Input: part model. Units: mm. Frame: model coordinates. Give positions to 0.01 mm unless a question says otherwise; leave off trailing zeros. Order: outer loops, then holes, each group sorted by start corner. A loop starts at its lowest first (then second) coordinate and runs counter-clockwise, first axis right, second up. Notation, with made-up numbers: (14.25, -11.5) -> (52.25, -11.5) arc R24 cw to (52.25, 17.5) -> close; hole circle Ø1 at (62, 41.25). An arc over 180 degrees is marked (long way). Use a Markdown table: item, result. Add a question column.
from build123d import *

# Parameters (mm, degrees)
F0_R     = 7.1501
F0_R_2   = 6.227401
F1_DEPTH = 4.7498


with BuildPart() as f1:
    # F0 (on Front) → F1 (new body)
    with BuildSketch(Plane.XZ):
        with BuildLine():
            Line((-139.7, -25.4), (139.7, -25.4))
            ThreePointArc((139.7, -25.4), (162.15064, -16.10064), (171.45, 6.35))
            Line((171.45, 6.35), (171.45, 19.05))
            ThreePointArc((171.45, 19.05), (169.590128, 23.540128), (165.1, 25.4))
            Line((165.1, 25.4), (-165.1, 25.4))
            ThreePointArc((-165.1, 25.4), (-169.590128, 23.540128), (-171.45, 19.05))
            Line((-171.45, 19.05), (-171.45, 6.35))
            ThreePointArc((-171.45, 6.35), (-162.15064, -16.10064), (-139.7, -25.4))
        make_face()
        with Locations((-101.6, -12.7)):
            Circle(F0_R, mode=Mode.SUBTRACT)
        with Locations((101.6, -12.7)):
            Circle(F0_R, mode=Mode.SUBTRACT)
        with Locations((-152.4, 7.62)):
            Circle(F0_R_2, mode=Mode.SUBTRACT)
        with Locations((152.4, 7.62)):
            Circle(F0_R_2, mode=Mode.SUBTRACT)
    extrude(amount=F1_DEPTH)


solid = f1.part
Q1. Ray query, line 1 (X direction, y = -0.4, z = 3); line 2 (X direction, y = -2.2, z = -13.5); line 3 (Z direction, x = -101.6, y = -2.8). Return the intervals inside material, ascending.
Q2. Section query A-A (y = -3.2). Return loops of the section in (x, z), plus the area to 3 significant figures.
Q3. Section query D-D (x = 152.4). Return loops of the section in (y, z).
Q4. Section query B-B (x = 101.6). Return loops of the section in (y, z), plus the area to 3 significant figures.
Q5. Draft query along X for faces 1 (the cylindrical face through (-169.54, -2.34, 23.59)), 2 (the flat face through (-2, -4.75, 0)), 3 (the cylindrical face through (-94.78, -2.34, -10.55)). Return one class per face: +X half, -X half, draft (parallel to the pull), parting line (faces both ways), or undercut.
Q6. Section query C-C (z = -9). Return loops of the section in (x, y), plus the area to 3 significant figures.
Q7. First-contact query: pin 1 (2 mm diameter, centred on y = -2, z = -14.5, fed in from -X). Flat tip, straight axial feed; report the tip coordinate or a pass-through.
Solution:
| question | item | result |
|---|---|---|
| 1 | line 1 | x = -171.27 to -156.58, -148.22 to 148.22, 156.58 to 171.27 |
| 1 | line 2 | x = -164.48 to -108.71, -94.49 to 94.49, 108.71 to 164.48 |
| 1 | line 3 | z = -25.4 to -19.85, -5.55 to 25.4 |
| 2 | outline | (-171.45, 6.35) arc R31.75 ccw to (-139.7, -25.4) -> (139.7, -25.4) arc R31.75 ccw to (171.45, 6.35) -> (171.45, 19.05) arc R6.35 ccw to (165.1, 25.4) -> (-165.1, 25.4) arc R6.35 ccw to (-171.45, 19.05) -> close; hole circle Ø12.45 at (-152.4, 7.62); hole circle Ø14.3 at (-101.6, -12.7); hole circle Ø14.3 at (101.6, -12.7); hole circle Ø12.45 at (152.4, 7.62) |
| 2 | area | 16,400 mm² |
| 3 | outline | (-4.75, -22.75) -> (0, -22.75) -> (0, 1.39) -> (-4.75, 1.39) -> close; (-4.75, 13.85) -> (0, 13.85) -> (0, 25.4) -> (-4.75, 25.4) -> close |
| 4 | outline | (-4.75, -25.4) -> (0, -25.4) -> (0, -19.85) -> (-4.75, -19.85) -> close; (-4.75, -5.55) -> (0, -5.55) -> (0, 25.4) -> (-4.75, 25.4) -> close |
| 4 | area | 173 mm² |
| 5 | face 1 | -X half |
| 5 | face 2 | draft |
| 5 | face 3 | undercut |
| 6 | outline | (-167.49, -4.75) -> (-107.72, -4.75) -> (-107.72, 0) -> (-167.49, 0) -> close; (-95.48, -4.75) -> (95.48, -4.75) -> (95.48, 0) -> (-95.48, 0) -> close; (107.72, -4.75) -> (167.49, -4.75) -> (167.49, 0) -> (107.72, 0) -> close |
| 6 | area | 1,470 mm² |
| 7 | pin 1 | stops at x = -164.48 |
